```python
from build123d import *

# Parameters (mm, degrees)
F1_DEPTH = 1.5875


# Not quite as in the source:
# - ends of sketch curves that miss each other by under 0.0002 mm in the source are joined


with BuildPart() as f1:
    # F0 (on Front) → F1 (new body)
    with BuildSketch(Plane.XZ):
        with BuildLine():
            Line((97.284460747, 47.1963935311), (-96.390539253, 47.1963935311))
            ThreePointArc((-96.390539253, 47.1963935311), (-105.370795374, 43.4766496521), (-109.090539253, 34.4963935311))
            Line((-109.090539253, 34.4963935311), (-109.090539253, -92.5036064689))
            Line((-109.090539253, -92.5036064689), (109.984460747, -92.5036064689))
            Line((109.984460747, -92.5036064689), (109.984460747, 34.4963935311))
            ThreePointArc((109.984460747, 34.4963935311), (106.2647168681, 43.4766496521), (97.284460747, 47.1963935311))
        make_face()
        with BuildLine():
            ThreePointArc((-53.3636475136, -45.7096316546), (-62.7650367506, -46.2093108693), (-62.3307099384, -36.8046758885))
            Line((-62.3307099384, -36.8046758885), (-9.0114088008, 16.8864949952))
            ThreePointArc((-9.0114088008, 16.8864949952), (4.2539e-06, 20.6375), (9.0114147958, 16.8864889585))
            Line((9.0114147958, 16.8864889585), (61.8517940181, -36.4462340741))
            ThreePointArc((61.8517940181, -36.4462340741), (63.9001946683, -38.7279945788), (64.640539253, -41.7036064689))
            ThreePointArc((64.640539253, -41.7036064689), (60.4161847378, -47.6872618127), (53.3636475136, -45.7096316546))
            Line((53.3636475136, -45.7096316546), (3.8656210952, -7.7286783496))
            ThreePointArc((3.8656210952, -7.7286783496), (0, -6.4164827869), (-3.8656210952, -7.7286783496))
            Line((-3.8656210952, -7.7286783496), (-53.3636475136, -45.7096316546))
        make_face(mode=Mode.SUBTRACT)
    extrude(amount=F1_DEPTH)


solid = f1.part
```
CAD build for the part. Positions are in the model's coordinates, mm. A direction names the side the tool comes from. Round coordinates to 2 decimals unless told otherwise and drop trailing zeros. Loops run counter-clockwise (first coordinate to the right, second up) from the corner with the lowest first, then second, coordinate; pieces in that order, holes last. Notation, with made-up numbers: (41.5, 59.25) - (89.5, 59.25) arc R19 ccw to (89.5, 80.25) - close; hole circle Ø9 at (-4, 20.25). An arc over 180 degrees is marked (long way). Return JSON: item names as keys, results as strings. Group by question number.
Q1. Band-saw the part on B-B on x = -21. Give the cut face in (y, z), plus the area to 3 significant figures.
Q2. Drill centre lines: line 1 along X through (y, z) = (-1.35, -22.5); line 2 along X through (y, z) = (-0.4, -14); line 3 along X through (y, z) = (-0.3, 6). Where is each one in solid material? Low to high. Write a range as [from, to].
Q3. Tool access for faces 1 (the face through (-36.04, -0.78, -10.33)), 2 (the face through (-1, -1.588, -22)): list every direction of +Z, -Z, +X, -X, +Y, -Y with a clear straight run to the whole face (end or side of a thin tool).
Q4. Band-saw the part on A-A on y = -1.1. Give the cut face in (x, z).
Q5. Band-saw the part on D-D on x = 57. Give the cut face in (y, z), plus the area to 3 significant figures.
Q6. Two-plate mould, pull along X, no slides. Class faces 3 (the face through (-105.272, -0.783, 43.575)), 4 (the face through (-28.268, -0.783, -26.453)), 5 (the face through (106.36, -0.78, 43.38)): +X half, -X half, draft (parallel to the pull), parting line (faces both ways), or undercut.
Q7. Band-saw the part on C-C on z = -28. Give the cut face in (x, y).
Solutions:
{
 "1": {"outline": "(-1.59, -92.5) - (0, -92.5) - (0, -20.88) - (-1.59, -20.88) - close; (-1.59, 4.81) - (0, 4.81) - (0, 47.2) - (-1.59, 47.2) - close", "area": "181 mm^2"},
 "2": {"line 1": "x = [-109.09, -48.13], [-23.12, 23.12], [48.03, 109.98]", "line 2": "x = [-109.09, -39.68], [-12.04, 12.04], [39.61, 109.98]", "line 3": "x = [-109.09, -19.82], [19.8, 109.98]"},
 "3": {"face 1": "+Y, -Y", "face 2": "+Z, -Z, +X, -X, -Y"},
 "4": {"outline": "(-109.09, -92.5) - (109.98, -92.5) - (109.98, 34.5) arc R12.7 ccw to (97.28, 47.2) - (-96.39, 47.2) arc R12.7 ccw to (-109.09, 34.5) - close; hole (-62.33, -36.8) arc R6.35 ccw (long way) to (-53.36, -45.71) - (-3.87, -7.73) arc R6.35 cw to (3.87, -7.73) - (53.36, -45.71) arc R6.35 ccw (long way) to (61.85, -36.45) - (9.01, 16.89) arc R12.7 ccw to (-9.01, 16.89) - close"},
 "5": {"outline": "(-1.59, -92.5) - (0, -92.5) - (0, -47.92) - (-1.59, -47.92) - close; (-1.59, -31.55) - (0, -31.55) - (0, 47.2) - (-1.59, 47.2) - close", "area": "196 mm^2"},
 "6": {"face 3": "-X half", "face 4": "undercut", "face 5": "+X half"},
 "7": {"outline": "(-109.09, -1.59) - (-53.59, -1.59) - (-53.59, 0) - (-109.09, 0) - close; (-30.28, -1.59) - (30.28, -1.59) - (30.28, 0) - (-30.28, 0) - close; (53.48, -1.59) - (109.98, -1.59) - (109.98, 0) - (53.48, 0) - close"}
}
